Geometry: see drawing. Coordinates: mm, zero at the bounding-box minimum. Round coordinates to 2 decimals unless told otherwise and drop trailing zeros. Loops run counter-clockwise (first coordinate to the right, second up) from the corner with the lowest first, then second, coordinate; pieces in that order, holes last. Notation, with made-up numbers: (32, 77.25) - (77, 77.25) arc R14 ccw to (77, 83.25) - close; hole circle Ø6 at (70.5, -28). An arc over 180 degrees is marked (long way). Use CSV: the item, a comma, the result in double quotes.
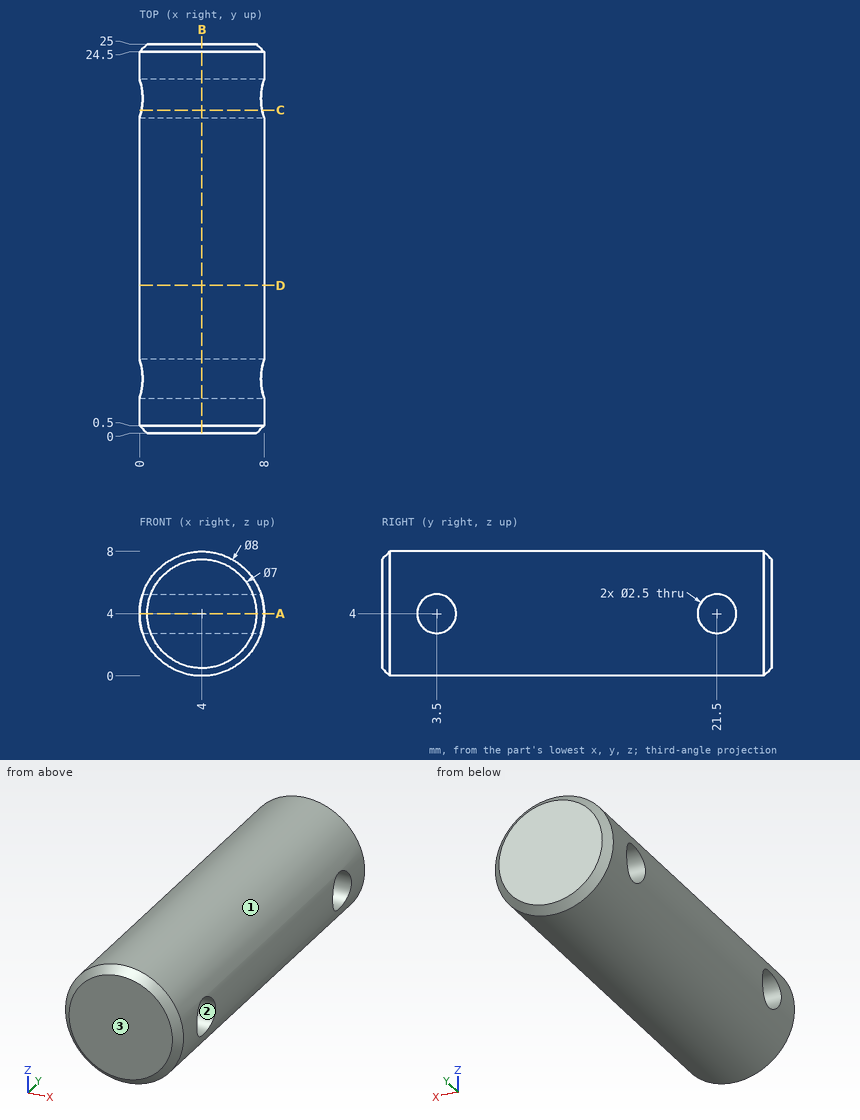
Item 1: Mould query, pull axis Z, two halves, no side actions, for the marked faces 1, 2 and 3. Classes: released by +Z, released by -Z, zero draft, split by the parting line, or undercut.
Final values:
face 1,"split by the parting line"
face 2,"undercut"
face 3,"zero draft"
Item 2: Material intervals for line 1 (Y direction, x = 0.5, z = 4.25); line 2 (Y direction, x = 7.75, z = 4.25); line 3 (X direction, y = 1.5, z = 5), sorted ascending.
Final values:
line 1,"y = 0.01 to 2.28, 4.72 to 20.28, 22.72 to 24.99"
line 2,"y = 0.26 to 2.28, 4.72 to 20.28, 22.72 to 24.74"
line 3,"x = 0.13 to 7.87"
Item 3: Section C-C on y = 20.75. Return the cut outline in (x, z), plus the area to 3 significant figures.
Final values:
outline,"(0.13, 3) arc R4 ccw to (7.87, 3) - close; (0.13, 5) - (7.87, 5) arc R4 ccw to start"
area,"34.4 mm²"
Item 4: Section B-B on x = 4. Return the cut outline in (y, z), plus the area to 3 significant figures.
Final values:
outline,"(0, 0.5) - (0.5, 0) - (24.5, 0) - (25, 0.5) - (25, 7.5) - (24.5, 8) - (0.5, 8) - (0, 7.5) - close; hole circle Ø2.5 at (3.5, 4); hole circle Ø2.5 at (21.5, 4)"
area,"190 mm²"
Item 5: Pin query (flat end, axial travel): P1, Ø2, axis at y = 21.5, z = 4, coming from the +X side; P2, Ø2, axis at y = 6.5, z = 5.5, coming from the -X side; P3, Ø3, axis at x = 6, y = 10, coming from the -Z side. Return the tip coordinate at first contact, or that it passes through.
Final values:
P1,"passes through"
P2,"stops at x = 0.03"
P3,"stops at z = 0.03"
Item 6: Section D-D on y = 9.5. Return the cut outline in (x, z), plus the area to 3 significant figures.
Final values:
outline,"circle Ø8 at (4, 4)"
area,"50.3 mm²"
Item 7: Section A-A on z = 4. Return the cut outline in (x, y), plus the area to 4 significant figures.
Final values:
outline,"(0, 0.5) - (0.5, 0) - (7.5, 0) - (8, 0.5) - (8, 2.25) - (0, 2.25) - close; (0, 4.75) - (8, 4.75) - (8, 20.25) - (0, 20.25) - close; (0, 22.75) - (8, 22.75) - (8, 24.5) - (7.5, 25) - (0.5, 25) - (0, 24.5) - close"
area,"159.5 mm²"
